```python
from build123d import *

# Parameters (mm, degrees)
SKETCH1_W            = 50
SKETCH1_H            = 40
BOSS_EXTRUDE1_DEPTH  = 3
SKETCH2_W            = 4
SKETCH2_H            = 40
BOSS_EXTRUDE2_DEPTH  = 24
SKETCH3_W            = 40
SKETCH3_H            = 13
CUT_EXTRUDE1_DEPTH   = 2
SKETCH5_W            = 2
SKETCH5_H            = 40
BOSS_EXTRUDE3_DEPTH  = 24
SKETCH6_R            = 2
CUT_EXTRUDE9_DEPTH   = 5
BOSS_EXTRUDE5_DEPTH  = 2
BOSS_EXTRUDE6_DEPTH  = 2
SKETCH12_W           = 44
SKETCH12_H           = 27
BOSS_EXTRUDE7_DEPTH  = 1
SKETCH14_W           = 44
SKETCH14_H           = 2
BOSS_EXTRUDE8_DEPTH  = 3
BOSS_EXTRUDE9_DEPTH  = 0.5
SKETCH15_W           = 44
SKETCH15_H           = 2
BOSS_EXTRUDE10_DEPTH = 3
SKETCH16_W           = 14.8
SKETCH16_H           = 3
CUT_EXTRUDE10_DEPTH  = 0.5
SKETCH17_W           = 44
SKETCH17_H           = 27
BOSS_EXTRUDE11_DEPTH = 4
SKETCH18_W           = 44
SKETCH18_H           = 24
CUT_EXTRUDE11_DEPTH  = 4
SKETCH21_R           = 14.25
CUT_EXTRUDE15_DEPTH  = 4
CUT_EXTRUDE16_START  = -4
CUT_EXTRUDE16_DEPTH  = 4
SKETCH24_W           = 44
SKETCH24_H           = 27
BOSS_EXTRUDE13_DEPTH = 1
SKETCH25_W           = 44
SKETCH25_H           = 12.5
CUT_EXTRUDE17_DEPTH  = 1
SKETCH26_W           = 44
SKETCH26_H           = 2
CUT_EXTRUDE18_DEPTH  = 1
SKETCH27_W           = 44
SKETCH27_H           = 2
CUT_EXTRUDE19_DEPTH  = 1
SKETCH28_W           = 44
SKETCH28_H           = 7.5
CUT_EXTRUDE20_DEPTH  = 3
SKETCH29_W           = 44
SKETCH29_H           = 27
BOSS_EXTRUDE14_DEPTH = 0.5


with BuildPart() as part:
    # Sketch1 → Boss-Extrude1 (new body)
    with BuildSketch(Plane(origin=(0, 0, 0), x_dir=(1, 0, 0), z_dir=(0, 1, 0))):
        with Locations((1.920937393, -5.615172506)):
            Rectangle(SKETCH1_W, SKETCH1_H)
    extrude(amount=BOSS_EXTRUDE1_DEPTH)

    # Sketch2 → Boss-Extrude2 (add)
    with BuildSketch(Plane(origin=(0, 3, 0), x_dir=(1, 0, 0), z_dir=(0, 1, 0))):
        with Locations((-21.079062607, -5.615172506)):
            Rectangle(SKETCH2_W, SKETCH2_H)
    extrude(amount=BOSS_EXTRUDE2_DEPTH)

    # Sketch3 → Cut-Extrude1 (cut)
    with BuildSketch(Plane(origin=(-19.079062607, 0, 0), x_dir=(0, 0, -1), z_dir=(1, 0, 0))):
        with Locations((-5.615172506, 18.5)):
            Rectangle(SKETCH3_W, SKETCH3_H)
    extrude(amount=-CUT_EXTRUDE1_DEPTH, mode=Mode.SUBTRACT)

    # Sketch5 → Boss-Extrude3 (add)
    with BuildSketch(Plane(origin=(0, 3, 0), x_dir=(1, 0, 0), z_dir=(0, 1, 0))):
        with Locations((25.920937393, -5.615172506)):
            Rectangle(SKETCH5_W, SKETCH5_H)
    extrude(amount=BOSS_EXTRUDE3_DEPTH)

    # Sketch6 → Cut-Extrude9 (cut)
    with BuildSketch(Plane.XZ):
        with Locations(Location((6.920937393, 23.115172506, 0), (0, 0, 270))):
            Circle(SKETCH6_R)
        with Locations(Location((6.920937393, -11.884827494, 0), (0, 0, 270))):
            Circle(SKETCH6_R)
        with BuildLine():
            Line((24.420937393, 13.015172506), (18.923020545, 13.015172506))
            ThreePointArc((18.923020545, 13.015172506), (-7.179062607, 5.615172506), (18.923020545, -1.784827494))
            Line((18.923020545, -1.784827494), (24.420937393, -1.784827494))
            Line((24.420937393, -1.784827494), (24.420937393, 5.615172506))
            Line((24.420937393, 5.615172506), (24.420937393, 13.015172506))
        make_face()
    extrude(amount=-CUT_EXTRUDE9_DEPTH, mode=Mode.SUBTRACT)

    # Sketch10 → Boss-Extrude5 (add)
    with BuildSketch(Plane.XY.offset(25.615172506)):
        Polygon((-19.079062607, 27), (-19.079062607, 25), (-21.079062607, 25), (-21.079062607, 12), (-19.079062607, 12), (-19.079062607, 3), (24.920937393, 3), (24.920937393, 27), (26.920937393, 27), (26.920937393, 0), (-23.079062607, 0), (-23.079062607, 27), align=None)
    extrude(amount=BOSS_EXTRUDE5_DEPTH)

    # Sketch11 → Boss-Extrude6 (add)
    with BuildSketch(Plane(origin=(0, 0, -14.384827494), x_dir=(-1, 0, 0), z_dir=(0, 0, -1))):
        Polygon((-26.920937393, 27), (-24.920937393, 27), (-24.920937393, 3), (19.079062607, 3), (19.079062607, 12), (21.079062607, 12), (21.079062607, 25), (19.079062607, 25), (19.079062607, 27), (23.079062607, 27), (23.079062607, 0), (-26.920937393, 0), align=None)
    extrude(amount=BOSS_EXTRUDE6_DEPTH)

    # Sketch12 → Boss-Extrude7 (add)
    with BuildSketch(Plane(origin=(26.920937393, 0, 0), x_dir=(0, 0, -1), z_dir=(1, 0, 0))):
        with Locations((-5.615172506, 13.5)):
            Rectangle(SKETCH12_W, SKETCH12_H)
    extrude(amount=BOSS_EXTRUDE7_DEPTH)

    # Sketch14 → Boss-Extrude8 (add)
    with BuildSketch(Plane(origin=(-19.079062607, 0, 0), x_dir=(0, 0, -1), z_dir=(1, 0, 0))):
        with Locations((-5.615172506, 26)):
            Rectangle(SKETCH14_W, SKETCH14_H)
    extrude(amount=BOSS_EXTRUDE8_DEPTH)

    # 3DSketch1 → Boss-Extrude9 (add)
    with BuildSketch(Plane(origin=(-21.079062607, 12, 27.615172506), x_dir=(0.04540766091864994, 0, -0.9989685402102996), z_dir=(0, -1, 0))):
        Polygon((0, 0), (0.090815322, 1.99793708), (44.045431091, 0), (43.954615769, -1.99793708), align=None)
    extrude(amount=-BOSS_EXTRUDE9_DEPTH)

    # Sketch15 → Boss-Extrude10 (add)
    with BuildSketch(Plane(origin=(-19.079062607, 0, 0), x_dir=(0, 0, -1), z_dir=(1, 0, 0))):
        with Locations((-5.615172506, 11.5)):
            Rectangle(SKETCH15_W, SKETCH15_H)
    extrude(amount=BOSS_EXTRUDE10_DEPTH)

    # Sketch16 → Cut-Extrude10 (cut)
    with BuildSketch(Plane.ZY.offset(-24.420937393)):
        with Locations((5.615172506, 1.5)):
            Rectangle(SKETCH16_W, SKETCH16_H)
    extrude(amount=-CUT_EXTRUDE10_DEPTH, mode=Mode.SUBTRACT)

    # Sketch17 → Boss-Extrude11 (add)
    with BuildSketch(Plane(origin=(27.920937393, 0, 0), x_dir=(0, 0, -1), z_dir=(1, 0, 0))):
        with Locations((-5.615172506, 13.5)):
            Rectangle(SKETCH17_W, SKETCH17_H)
    extrude(amount=BOSS_EXTRUDE11_DEPTH)

    # Sketch18 → Cut-Extrude11 (cut)
    with BuildSketch(Plane.ZY.offset(-24.920937393)):
        with Locations((5.615172506, 15)):
            Rectangle(SKETCH18_W, SKETCH18_H)
    extrude(amount=-CUT_EXTRUDE11_DEPTH, mode=Mode.SUBTRACT)

    # Sketch21 → Cut-Extrude15 (cut)
    with BuildSketch(Plane(origin=(0, 0, 0), x_dir=(-1, 0, 0), z_dir=(0, -1, 0))):
        with Locations((-6.920937393, -5.615172506)):
            Circle(SKETCH21_R)
    extrude(amount=-CUT_EXTRUDE15_DEPTH, mode=Mode.SUBTRACT)

    # Sketch22 → Cut-Extrude16 (cut)
    with BuildSketch(Plane(origin=(0, 3, 0), x_dir=(1, 0, 0), z_dir=(0, 1, 0)).offset(CUT_EXTRUDE16_START)):
        with BuildLine():
            ThreePointArc((21.106680727, 1.784827494), (20.39103932, 3.019158274), (19.568281538, 4.184827494))
            Line((19.568281538, 4.184827494), (17.266105347, 4.184827494))
            ThreePointArc((17.266105347, 4.184827494), (18.246250908, 3.03351374), (19.09888878, 1.784827494))
            Line((19.09888878, 1.784827494), (21.106680727, 1.784827494))
        make_face()
        with BuildLine():
            Line((17.266105347, -15.415172506), (19.568281538, -15.415172506))
            ThreePointArc((19.568281538, -15.415172506), (20.39103932, -14.249503286), (21.106680727, -13.015172506))
            Line((21.106680727, -13.015172506), (19.09888878, -13.015172506))
            ThreePointArc((19.09888878, -13.015172506), (18.246250908, -14.263858752), (17.266105347, -15.415172506))
        make_face()
    extrude(amount=CUT_EXTRUDE16_DEPTH, mode=Mode.SUBTRACT)

    # Sketch24 → Boss-Extrude13 (add)
    with BuildSketch(Plane.ZY.offset(23.079062607)):
        with Locations((5.615172506, 13.5)):
            Rectangle(SKETCH24_W, SKETCH24_H)
    extrude(amount=BOSS_EXTRUDE13_DEPTH)

    # Sketch25 → Cut-Extrude17 (cut)
    with BuildSketch(Plane(origin=(-21.079062607, 0, 0), x_dir=(0, 0, -1), z_dir=(1, 0, 0))):
        with Locations((-5.615172506, 18.75)):
            Rectangle(SKETCH25_W, SKETCH25_H)
    extrude(amount=-CUT_EXTRUDE17_DEPTH, mode=Mode.SUBTRACT)

    # Sketch26 → Cut-Extrude18 (cut)
    with BuildSketch(Plane(origin=(-16.079062607, 0, 0), x_dir=(0, 0, -1), z_dir=(1, 0, 0))):
        with Locations((-5.615172506, 26)):
            Rectangle(SKETCH26_W, SKETCH26_H)
    extrude(amount=-CUT_EXTRUDE18_DEPTH, mode=Mode.SUBTRACT)

    # Sketch27 → Cut-Extrude19 (cut)
    with BuildSketch(Plane(origin=(-16.079062607, 0, 0), x_dir=(0, 0, -1), z_dir=(1, 0, 0))):
        with Locations((-5.615172506, 11.5)):
            Rectangle(SKETCH27_W, SKETCH27_H)
    extrude(amount=-CUT_EXTRUDE19_DEPTH, mode=Mode.SUBTRACT)

    # Sketch28 → Cut-Extrude20 (cut)
    with BuildSketch(Plane(origin=(-19.079062607, 0, 0), x_dir=(0, 0, -1), z_dir=(1, 0, 0))):
        with Locations((-5.615172506, 6.75)):
            Rectangle(SKETCH28_W, SKETCH28_H)
    extrude(amount=-CUT_EXTRUDE20_DEPTH, mode=Mode.SUBTRACT)

    # Sketch29 → Boss-Extrude14 (add)
    with BuildSketch(Plane.ZY.offset(24.079062607)):
        with Locations((5.615172506, 13.5)):
            Rectangle(SKETCH29_W, SKETCH29_H)
    extrude(amount=BOSS_EXTRUDE14_DEPTH)


solid = part.part
```
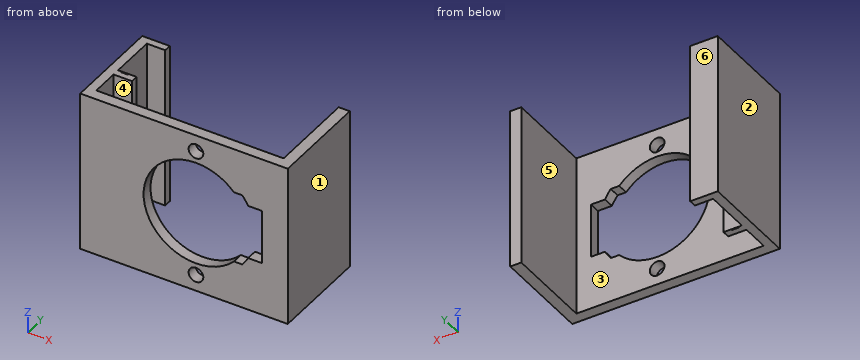
Read the model definition and answer for the solid it produces. Units are mm, in the model's axes. Face numbers are marked on the shaded views. A direction names the side the tool comes from. Give positions to 0.01 mm unless a question says otherwise; leave off trailing zeros. Loops run counter-clockwise (first coordinate to the right, second up) from the corner with the lowest first, then second, coordinate; pieces in that order, holes last.
Item 1: The part is cut by section B-B (x = 22.5). Write down the section's boundary in (y, z), and give its area (3 significant figures).
Item 2: The part is cut by section A-A (y = 24.25). Write down the section's boundary in (x, z), and give its area (3 significant figures).
Item 3: The part is cut by section D-D (z = 3). Write down the section's boundary in (x, y).
Item 4: Each of these flat-tipped pins is pushed along its axis until it touches: pin 1 Ø1 at (x, y) = (-16.5, 14.5) entering from -Z; pin 2 Ø8 at (x, z) = (-13, 15.5) entering from +Y. Where does it stop, or does it pass through?
Item 5: Find the intervals of material crossed by line 1 along Y through (x, z) = (-21.5, 20); line 2 along X through (y, z) = (17.25, 8.5); line 3 along Y through (x, z) = (25.5, 12.5), in increasing order.
Item 6: The mould has two halves that part along X. Classify the marked faces 1, 2 and 3: released by +X, released by -X, zero draft, split by the parting line, or undercut.
Item 7: For the marked faces 4, 5 and 6, determine the directions among +Z, -Z, +X, -X, +Y, -Y from which every point of the face is accessible in a straight line to the end or side of a thin tool.
Item 8: The part is cut by section C-C (x = 8). Write down the section's boundary in (y, z).
Taken from the geometry:
1. outline: (0, -16.38) - (3, -16.38) - (3, -1.78) - (0, -1.78) - close; (0, 13.02) - (3, 13.02) - (3, 27.62) - (0, 27.62) - close
1. area: 87.6 mm2
2. outline: (-24.58, -16.38) - (-22.08, -16.38) - (-22.08, 27.62) - (-24.58, 27.62) - close; (28.92, -16.38) - (31.92, -16.38) - (31.92, 27.62) - (28.92, 27.62) - close
2. area: 242 mm2
3. outline: (-24.58, 0) - (-7.09, 0) - (-7.09, 3) - (-22.08, 3) - (-22.08, 10.5) - (-17.08, 10.5) - (-17.08, 12.5) - (-22.08, 12.5) - (-22.08, 25) - (-17.08, 25) - (-17.08, 27) - (-24.58, 27) - close; (24.92, 0) - (31.92, 0) - (31.92, 27) - (28.92, 27) - (28.92, 3) - (24.92, 3) - close
4. pin 1: passes through
4. pin 2: stops at y = 3
5. line 1: y = 0 to 3, 10.5 to 12.5, 25 to 27
5. line 2: x = -24.58 to -22.08, 28.92 to 31.92
5. line 3: y = 0 to 3
6. face 1: released by +X
6. face 2: released by -X
6. face 3: undercut
7. face 4: +Z, -Z
7. face 5: +Z, -Z, +Y
7. face 6: +Z, -Z, +X, -X, +Y
8. outline: (0, -16.38) - (3, -16.38) - (3, -13.57) - (0, -13.57) - close; (0, -10.2) - (3, -10.2) - (3, -8.59) - (0, -8.59) - close; (0, 19.82) - (3, 19.82) - (3, 21.43) - (0, 21.43) - close; (0, 24.8) - (3, 24.8) - (3, 27.62) - (0, 27.62) - close
